Read the model definition and answer for the solid it produces. Units are mm, in the model's axes. A direction names the side the tool comes from. Coordinates: 2 decimals unless noted, no trailing zeros. Write each loop counter-clockwise with the first axis right and the second up, starting at its lowest first coordinate (ties: lowest second). Pieces come first, ordered by that corner, then holes. Notation, with made-up numbers: (57, 21) -> (86, 21) arc R14 ccw to (86, 26) -> close; hole circle Ø2 at (88.25, 66). An arc over 180 degrees is marked (long way). Answer as a JSON object with one key per item and string values. Group by question number.
(1) Find section D-D (z = -7). Give the vertices of the cut face in (x, y), then the cut area to 3 significant figures.
(2) Find section B-B (y = 6). Give the vertices of the cut face in (x, z).
(3) Straight lines are drawn through the part: L1, parallel to X at y = 1, z = -13; L2, parallel to Z at x = 5.5, y = 4.5; L3, parallel to Y at x = 5.25, z = -1. For each, find the intervals that lie inside material, in ascending order.
(4) Which of the six approach directions +Z, -Z, +X, -X, +Y, -Y give full straight-line access (tool end or side, diameter ignored) to faces 4 (the face through (-0.2, 0.4, 19)), 5 (the face through (-12, 5, 16.5)), 6 (the face through (-5, 4.2, -18.5)), 7 (the face through (-8, 4, 18)), 8 (the face through (12, 4, -3))?
(5) Find section A-A (y = 4.25). Count the separate pieces of the cut face and the enclosed holes in it, then the cut area to 3 significant figures.
(6) Find section C-C (x = 6.25). Give the vertices of the cut face in (y, z), then the cut area to 3 significant figures.
(7) Flat-ended cylindrical pins translate along their axes: P1, Ø0.5, axis at x = -12, z = 0.5, coming from the -Y side; P2, Ø0.8, axis at x = 12, z = -17, coming from the +Y side. Find the tip coordinate at first contact, or state that the pin passes through.
(8) For a pull along Y with two mould halves and no side action, classify faces 1 (the face through (-0.2, 0.4, -19)), 2 (the face through (12, 5, 0)), 3 (the face through (0, 0, 0)) as +Y half, -Y half, draft (parallel to the pull), parting line (faces both ways), or undercut.
from build123d import *

# Parameters (mm, degrees)
SKETCH1_W               = 25
SKETCH1_H               = 38
BOSS_EXTRUDE1_DEPTH     = 7.6
SKETCH2_W               = 23
SKETCH2_H               = 36
CUT_EXTRUDE1_DEPTH      = 6.8
SKETCH2_3_W             = 1
SKETCH2_3_H             = 1.5
CUT_EXTRUDE2_DEPTH      = 5.6
CUT_EXTRUDE3_DEPTH      = 24.97936613
CUT_EXTRUDE3_DEPTH_BACK = 24.97936613
SKETCH3_W               = 6
SKETCH3_H               = 1.2
SKETCH4_W               = 6.5
SKETCH4_H               = 1
SKETCH4_W_2             = 10
CUT_EXTRUDE4_DEPTH      = 6.8


with BuildPart() as part:
    # Sketch1 → Boss-Extrude1 (new body)
    with BuildSketch(Plane(origin=(0, 0, 0), x_dir=(1, 0, 0), z_dir=(0, 1, 0))):
        Rectangle(SKETCH1_W, SKETCH1_H)
    extrude(amount=BOSS_EXTRUDE1_DEPTH)

    # Sketch2 → Cut-Extrude1 (cut)
    with BuildSketch(Plane(origin=(0, 7.6, 0), x_dir=(1, 0, 0), z_dir=(0, 1, 0))):
        Rectangle(SKETCH2_W, SKETCH2_H)
    extrude(amount=-CUT_EXTRUDE1_DEPTH, mode=Mode.SUBTRACT)

    # Sketch2<3> → Cut-Extrude2 (cut)
    with BuildSketch(Plane(origin=(0, 7.6, 0), x_dir=(1, 0, 0), z_dir=(0, 1, 0))):
        with Locations((-12, 17.25)):
            Rectangle(SKETCH2_3_W, SKETCH2_3_H)
        with Locations((12, 17.25)):
            Rectangle(SKETCH2_3_W, SKETCH2_3_H)
        with Locations((-12, -17.25)):
            Rectangle(SKETCH2_3_W, SKETCH2_3_H)
        with Locations((12, -17.25)):
            Rectangle(SKETCH2_3_W, SKETCH2_3_H)
    extrude(amount=-CUT_EXTRUDE2_DEPTH, mode=Mode.SUBTRACT)

    # Sketch3 → Cut-Extrude3 (cut, two sides: drawn at the far end of the back side and taken through both)
    with BuildSketch(Plane(origin=(0, 0, 0), x_dir=(0, 0, -1), z_dir=(1, 0, 0)).offset(-CUT_EXTRUDE3_DEPTH_BACK)):
        with Locations((0, 4.4)):
            Rectangle(SKETCH3_W, SKETCH3_H)
    extrude(amount=CUT_EXTRUDE3_DEPTH + CUT_EXTRUDE3_DEPTH_BACK, mode=Mode.SUBTRACT)

    # Sketch4 → Cut-Extrude4 (cut)
    with BuildSketch(Plane(origin=(0, 7.6, 0), x_dir=(1, 0, 0), z_dir=(0, 1, 0))):
        with Locations((0, -18.5)):
            Rectangle(SKETCH4_W, SKETCH4_H)
        with Locations((0, 18.5)):
            Rectangle(SKETCH4_W_2, SKETCH4_H)
    extrude(amount=-CUT_EXTRUDE4_DEPTH, mode=Mode.SUBTRACT)


solid = part.part
Results below:
{
 "1": {"outline": "(-12.5, 0) -> (12.5, 0) -> (12.5, 7.6) -> (11.5, 7.6) -> (11.5, 0.8) -> (-11.5, 0.8) -> (-11.5, 7.6) -> (-12.5, 7.6) -> close", "area": "33.6 mm2"},
 "2": {"outline": "(-12.5, -19) -> (-5, -19) -> (-5, -18) -> (-12.5, -18) -> close; (-12.5, -16.5) -> (-11.5, -16.5) -> (-11.5, 16.5) -> (-12.5, 16.5) -> close; (-12.5, 18) -> (-3.25, 18) -> (-3.25, 19) -> (-12.5, 19) -> close; (3.25, 18) -> (12.5, 18) -> (12.5, 19) -> (3.25, 19) -> close; (5, -19) -> (12.5, -19) -> (12.5, -18) -> (5, -18) -> close; (11.5, -16.5) -> (12.5, -16.5) -> (12.5, 16.5) -> (11.5, 16.5) -> close"},
 "3": {"L1": "x = -12.5 to -11.5, 11.5 to 12.5", "L2": "z = -19 to -18, 18 to 19", "L3": "y = 0 to 0.8"},
 "4": {"face 4": "+Z, +X, -X, +Y, -Y", "face 5": "+X, -X, +Y", "face 6": "-Z, +Y", "face 7": "+Y", "face 8": "+X, -X"},
 "5": {"separate pieces": "8", "enclosed holes": "0", "area": "87.5 mm2"},
 "6": {"outline": "(0, -19) -> (7.6, -19) -> (7.6, -18) -> (0.8, -18) -> (0.8, 18) -> (7.6, 18) -> (7.6, 19) -> (0, 19) -> close", "area": "44.0 mm2"},
 "7": {"P1": "stops at y = 0", "P2": "stops at y = 2"},
 "8": {"face 1": "draft", "face 2": "undercut", "face 3": "-Y half"}
}
